Geometry check sheet. Reference: the model listing, model coordinates, mm. Face numbers are marked on the shaded views. A direction names the side the tool comes from. Coordinates: 2 decimals unless noted, no trailing zeros. Write each loop counter-clockwise with the first axis right and the second up, starting at its lowest first coordinate (ties: lowest second). Pieces come first, ordered by that corner, then holes.
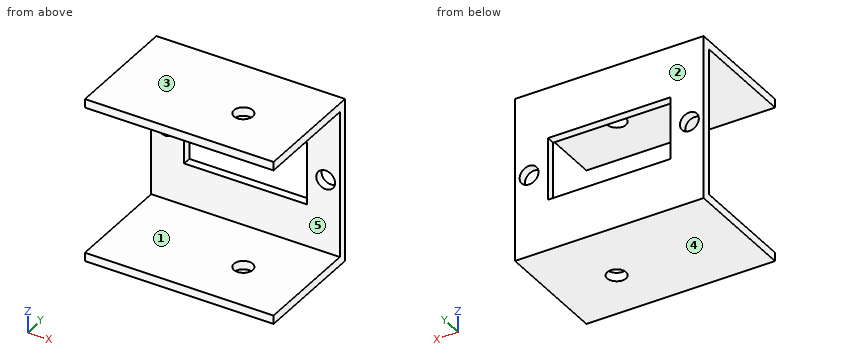
from build123d import *

# Parameters (mm, degrees)
SKETCH1_W           = 45
SKETCH1_H           = 30.48
SKETCH1_R           = 1.75
SKETCH1_W_2         = 22.75
SKETCH1_H_2         = 11.6
BOSS_EXTRUDE1_DEPTH = 1.59
SKETCH3_W           = 45
SKETCH3_H           = 1.59
BOSS_EXTRUDE3_DEPTH = 20
SKETCH4_R           = 1.75
CUT_EXTRUDE2_DEPTH  = 40
SKETCH5_W           = 5
SKETCH5_H           = 30.48
CUT_EXTRUDE3_DEPTH  = 30


with BuildPart() as part:
    # Sketch1 → Boss-Extrude1 (new body)
    with BuildSketch(Plane(origin=(0, 0, 0), x_dir=(1, 0, 0), z_dir=(0, 1, 0))):
        Rectangle(SKETCH1_W, SKETCH1_H)
        with Locations(Location((-14.875, 0, 0), (0, 0, 90))):
            Circle(SKETCH1_R, mode=Mode.SUBTRACT)
        with Locations(Location((14.875, 0, 0), (0, 0, 90))):
            Circle(SKETCH1_R, mode=Mode.SUBTRACT)
        Rectangle(SKETCH1_W_2, SKETCH1_H_2, mode=Mode.SUBTRACT)
    extrude(amount=BOSS_EXTRUDE1_DEPTH)

    # Sketch3 → Boss-Extrude3 (add)
    with BuildSketch(Plane(origin=(0, 0, 0), x_dir=(-1, 0, 0), z_dir=(0, -1, 0))):
        with Locations((0, -14.445)):
            Rectangle(SKETCH3_W, SKETCH3_H)
        with Locations((0, 14.445)):
            Rectangle(SKETCH3_W, SKETCH3_H)
    extrude(amount=BOSS_EXTRUDE3_DEPTH)

    # Sketch4 → Cut-Extrude2 (cut)
    with BuildSketch(Plane.XY.offset(15.24)):
        with Locations((6, -10.41)):
            Circle(SKETCH4_R)
    extrude(amount=-CUT_EXTRUDE2_DEPTH, mode=Mode.SUBTRACT)

    # Sketch5 → Cut-Extrude3 (cut)
    with BuildSketch(Plane(origin=(0, 1.59, 0), x_dir=(1, 0, 0), z_dir=(0, 1, 0))):
        with Locations((-20, 0)):
            Rectangle(SKETCH5_W, SKETCH5_H)
        with Locations((20, 0)):
            Rectangle(SKETCH5_W, SKETCH5_H)
    extrude(amount=-CUT_EXTRUDE3_DEPTH, mode=Mode.SUBTRACT)


solid = part.part
1. Sectioned sample at B-B, the plane x = 6. Record the boundary of the cut face in (y, z), and give its area (3 significant figures).
Computed values:
outline: (-20, -15.24) - (-12.16, -15.24) - (-12.16, -13.65) - (-20, -13.65) - close; (-20, 13.65) - (-12.16, 13.65) - (-12.16, 15.24) - (-20, 15.24) - close; (-8.66, -15.24) - (1.59, -15.24) - (1.59, -5.8) - (0, -5.8) - (0, -13.65) - (-8.66, -13.65) - close; (-8.66, 13.65) - (0, 13.65) - (0, 5.8) - (1.59, 5.8) - (1.59, 15.24) - (-8.66, 15.24) - close
area: 82.5 mm2
2. Gauge pin test, flat ends, axial feed: pin 1 Ø10 at (x, z) = (1.5, 0.5) entering from +Y; pin 2 Ø4.5 at (x, z) = (14.875, 0) entering from -Y. Record the tip position at first contact, or that the pin passes through.
Computed values:
pin 1: passes through
pin 2: stops at y = 0
3. Access from +Z, -Z, +X, -X, +Y, -Y to the whole of each face (thin tool, end or side, straight path). Record for the marked faces 1 and 2.
Computed values:
face 1: +X, -X, -Y
face 2: +Z, -Z, +X, -X, +Y
4. Draft check along Z on the marked faces 3, 4 and 5. Enter one of: released by +Z, released by -Z, zero draft, split by the parting line, or undercut.
Computed values:
face 3: released by +Z
face 4: released by -Z
face 5: undercut
5. Sectioned sample at A-A, the plane z = -3.5. Record the boundary of the cut face in (x, y) (3 decimals), and give its area (3 significant figures).
Computed values:
outline: (-17.5, 0) - (-11.375, 0) - (-11.375, 1.59) - (-17.5, 1.59) - close; (11.375, 0) - (17.5, 0) - (17.5, 1.59) - (11.375, 1.59) - close
area: 19.5 mm2
6. Sectioned sample at D-D, the plane z = 0. Record the boundary of the cut face in (x, y) (3 decimals).
Computed values:
outline: (-17.5, 0) - (-16.625, 0) - (-16.625, 1.59) - (-17.5, 1.59) - close; (-13.125, 0) - (-11.375, 0) - (-11.375, 1.59) - (-13.125, 1.59) - close; (11.375, 0) - (13.125, 0) - (13.125, 1.59) - (11.375, 1.59) - close; (16.625, 0) - (17.5, 0) - (17.5, 1.59) - (16.625, 1.59) - close
7. Thickness scan on line 1 along X through (y, z) = (1.05, 0) (3 decimals); line 2 along Z through (x, y) = (-6, -1); line 3 along Y through (x, z) = (6, 14). Record the ranges inside material, lowest first.
Computed values:
line 1: x = -17.5 to -16.625, -13.125 to -11.375, 11.375 to 13.125, 16.625 to 17.5
line 2: z = -15.24 to -13.65, 13.65 to 15.24
line 3: y = -20 to -12.16, -8.66 to 1.59
8. Sectioned sample at C-C, the plane y = -18.5. Record the boundary of the cut face in (x, z).
Computed values:
outline: (-17.5, -15.24) - (17.5, -15.24) - (17.5, -13.65) - (-17.5, -13.65) - close; (-17.5, 13.65) - (17.5, 13.65) - (17.5, 15.24) - (-17.5, 15.24) - close
